Could you check a few things on this model? Use its own coordinates, in mm. A direction names the side the tool comes from. Give positions to 0.01 mm unless a question says otherwise; leave off trailing zeros. Write each loop counter-clockwise with the first axis right and the second up, starting at its lowest first coordinate (ties: lowest second). Pieces come first, ordered by that corner, then holes. Notation, with made-up numbers: (24.25, 75) - (32.25, 75) arc R33 ccw to (32.25, 113) - close; hole circle Ø9 at (74.5, 68.5). An arc over 180 degrees is marked (long way). Use one line per item in the form item = value.
```python
from build123d import *

# Parameters (mm, degrees)
SKETCH1_R           = 30
SKETCH1_R_2         = 20
BOSS_EXTRUDE1_DEPTH = 3
SKETCH2_R           = 2.55
BOSS_EXTRUDE2_DEPTH = 3
CIRPATTERN1_COUNT   = 3
BOSS_EXTRUDE3_DEPTH = 3
SKETCH4_R           = 2.05
CUT_EXTRUDE1_DEPTH  = 104.489129864
SKETCH6_R           = 1.75
CUT_EXTRUDE2_DEPTH  = 104.489129864
CIRPATTERN2_COUNT   = 6
CUT_EXTRUDE3_DEPTH  = 104.489129864
FILLET1_R           = 5
FILLET2_R           = 6.5


with BuildPart() as part:
    # Sketch1 → Boss-Extrude1 (new body)
    with BuildSketch(Plane(origin=(0, 0, 0), x_dir=(1, 0, 0), z_dir=(0, 1, 0))):
        with Locations(Location((0, 0, 0), (0, 0, 270))):
            Circle(SKETCH1_R)
        with Locations(Location((0, 0, 0), (0, 0, 270))):
            Circle(SKETCH1_R_2, mode=Mode.SUBTRACT)
    extrude(amount=BOSS_EXTRUDE1_DEPTH)

    # Sketch2 → Boss-Extrude2 (add)
    with BuildSketch(Plane(origin=(0, 3, 0), x_dir=(1, 0, 0), z_dir=(0, 1, 0))):
        with BuildLine():
            Line((-4.75, 15.25), (-4.75, 19.42775077))
            ThreePointArc((-4.75, 19.42775077), (0, 20), (4.75, 19.42775077))
            Line((4.75, 19.42775077), (4.75, 15.25))
            ThreePointArc((4.75, 15.25), (0, 10.5), (-4.75, 15.25))
        make_face()
        with Locations(Location((0, 15.25, 0), (0, 0, 270))):
            Circle(SKETCH2_R, mode=Mode.SUBTRACT)
    boss_extrude2 = extrude(amount=-BOSS_EXTRUDE2_DEPTH)

    # CirPattern1: Boss-Extrude2 ×3 about axis
    cirpattern1_axis = Axis((0, 0, 0), (0, 1, 0))
    for i in range(1, CIRPATTERN1_COUNT):
        add(boss_extrude2.rotate(cirpattern1_axis, i * 360 / CIRPATTERN1_COUNT))

    # Sketch3 → Boss-Extrude3 (add)
    with BuildSketch(Plane(origin=(0, 3, 0), x_dir=(1, 0, 0), z_dir=(0, 1, 0))):
        with BuildLine():
            Line((20.396078054, 22), (99, 22))
            Line((99, 22), (99, 7))
            Line((99, 7), (29.171904292, 7))
            ThreePointArc((29.171904292, 7), (25.893941733, 15.149382216), (20.396078054, 22))
        make_face()
        with BuildLine():
            Line((29.171904292, -7), (99, -7))
            Line((99, -7), (99, -22))
            Line((99, -22), (20.396078054, -22))
            ThreePointArc((20.396078054, -22), (25.893941733, -15.149382216), (29.171904292, -7))
        make_face()
    extrude(amount=-BOSS_EXTRUDE3_DEPTH)

    # Sketch4 → Cut-Extrude1 (cut, through all)
    with BuildSketch(Plane(origin=(0, 3, 0), x_dir=(1, 0, 0), z_dir=(0, 1, 0))):
        with Locations(Location((54, 14.5, 0), (0, 0, 270))):
            Circle(SKETCH4_R)
        with Locations(Location((84, 14.5, 0), (0, 0, 270))):
            Circle(SKETCH4_R)
        with Locations(Location((54, -14.5, 0), (0, 0, 270))):
            Circle(SKETCH4_R)
        with Locations(Location((84, -14.5, 0), (0, 0, 270))):
            Circle(SKETCH4_R)
    extrude(amount=-CUT_EXTRUDE1_DEPTH, mode=Mode.SUBTRACT)

    # Sketch6 → Cut-Extrude2 (cut, through all)
    with BuildSketch(Plane.XZ):
        with Locations(Location((25, 0, 0), (0, 0, 270))):
            Circle(SKETCH6_R)
    cut_extrude2 = extrude(amount=-CUT_EXTRUDE2_DEPTH, mode=Mode.SUBTRACT)

    # CirPattern2: Cut-Extrude2 ×6 about axis
    cirpattern2_axis = Axis((0, 0, 0), (0, 1, 0))
    for i in range(1, CIRPATTERN2_COUNT):
        add(cut_extrude2.rotate(cirpattern2_axis, i * 360 / CIRPATTERN2_COUNT), mode=Mode.SUBTRACT)

    # Sketch7 → Cut-Extrude3 (cut, through all)
    with BuildSketch(Plane.XZ):
        with BuildLine():
            Line((99, 22), (84, 22))
            ThreePointArc((84, 22), (91.5, 14.5), (84, 7))
            Line((84, 7), (99, 7))
            Line((99, 7), (99, 22))
        make_face()
        with BuildLine():
            Line((99, -7), (84, -7))
            ThreePointArc((84, -7), (91.5, -14.5), (84, -22))
            Line((84, -22), (99, -22))
            Line((99, -22), (99, -7))
        make_face()
    extrude(amount=-CUT_EXTRUDE3_DEPTH, mode=Mode.SUBTRACT)

    # Fillet1
    fillet1_edges = [part.edges().sort_by_distance(p)[0] for p in [
        (19.199925706, 1.5, 5.600254717),
        (14.449925706, 1.5, 13.827496053),
        (-19.199925706, 1.5, 5.600254717),
        (-14.449925706, 1.5, 13.827496053),
        (4.75, 1.5, -19.42775077),
        (-4.75, 1.5, -19.42775077),
    ]]
    fillet(fillet1_edges, radius=FILLET1_R)

    # Fillet2
    fillet2_edges = [part.edges().sort_by_distance(p)[0] for p in [
        (29.171904292, 1.5, -7),
        (20.396078054, 1.5, -22),
        (20.396078054, 1.5, 22),
        (29.171904292, 1.5, 7),
    ]]
    fillet(fillet2_edges, radius=FILLET2_R)


solid = part.part
```
1. If I drill on line 1 (Z direction, x = 63.5, y = 2); line 2 (X direction, y = 0.75, z = -15.25); line 3 (Z direction, x = -11, y = 1.3), over which ranges is the centre line in solid material (lowest first)? Write a range as from..to.
Response values:
line_1 = -22..-7, 7..22
line_2 = -25.83..-12.94, -5.45..-2.55, 2.55..5.45, 12.94..52.09, 55.91..82.09, 85.91..91.46
line_3 = -27.91..-22.55, -20.75..-16.53, 3.42..6.35, 8.9..20.75, 22.55..27.91
2. Imagine slicing it at C-C, the plane z = 14.5. State how many separate pieces and enclosed holes the cut face has, and give its area (3 significant figures).
Response values:
separate_pieces = 4
enclosed_holes = 0
area = 265 mm²
3. Which directions (+Z, -Z, +X, -X, +Y, -Y) give clear straight access to the entire face, cutting with the end or side of a thin tool? Please do faces 1 (the face through (0, 1, 20)), 2 (the face through (61, 2, -7)), 3 (the face through (54, 2, 22)), 4 (the face through (32, 0, 6)).
Response values:
face_1 = +Y, -Y
face_2 = +X, +Y, -Y
face_3 = +Z, +X, +Y, -Y
face_4 = +Z, -Z, +X, -X, -Y
4. Imagine slicing it at D-D, the plane x = -25. List the corners of the cut face in (y, z) for me.
Response values:
outline = (0, -16.58) - (3, -16.58) - (3, -1.75) - (0, -1.75) - close; (0, 1.75) - (3, 1.75) - (3, 16.58) - (0, 16.58) - close
5. If we mould it in two halves opening along Z, with no side actions, what happens to faces 5 (the face through (32, 3, 6)), 6 (the face through (20.623, 1.479, -22.377)), 7 (the face through (56.033, 1.521, 14.233))? For each: pulls with the +Z half, pulls with the -Z half, needs draft (parallel to the pull), parting line crosses it, or undercut.
Response values:
face_5 = needs draft
face_6 = pulls with the -Z half
face_7 = undercut
6. Imagine slicing it at A-A, the plane x = 72.5. List the corners of the cut face in (y, z) for me.
Response values:
outline = (0, -22) - (3, -22) - (3, -7) - (0, -7) - close; (0, 7) - (3, 7) - (3, 22) - (0, 22) - close
7. Imagine slicing it at B-B, the plane x = 54. List the corners of the cut face in (y, z) for me.
Response values:
outline = (0, -22) - (3, -22) - (3, -16.55) - (0, -16.55) - close; (0, -12.45) - (3, -12.45) - (3, -7) - (0, -7) - close; (0, 7) - (3, 7) - (3, 12.45) - (0, 12.45) - close; (0, 16.55) - (3, 16.55) - (3, 22) - (0, 22) - close
8. For pin 1 (6.5 mm diameter, centred on x = 84, z = -14.5, fed in from -Y); pin 2 (1.5 mm diameter, centred on x = 45, y = 2, fed in from +Z); pin 3 (0.9 mm diameter, centred on x = 39, y = 2, fed in from -Z), each with a flat end and sliding along its axis, tell me the tip position at first contact or that it passes through.
Response values:
pin_1 = 0
pin_2 = 22
pin_3 = -22
